Model file for the job. Use its own axes, mm. Face numbers are marked on the shaded views. A direction names the side the tool comes from. Give positions to 0.01 mm unless a question says otherwise; leave off trailing zeros. Order: outer loops, then holes, each group sorted by start corner. A loop starts at its lowest first (then second) coordinate and runs counter-clockwise, first axis right, second up. Notation, with made-up numbers: (58, 8.25) - (106, 8.25) arc R16 ccw to (106, 38.25) - close; hole circle Ø8 at (40, 4). An arc over 180 degrees is marked (long way). Use CSV: the item, a comma, the result in double quotes. Start each with the question number.
(1) Band-saw the part on A-A, the plane x = 0. Count the separate pieces of the cut face and the enclosed holes in it, then the cut area to 3 significant figures.
(2) Probe L1, parallel to Y at x = 0, z = -0.5 (3 decimals); L2, parallel to Y at x = -0.25, z = -3.25 (3 decimals); L3, parallel to Z at x = 4, y = 29. List the from-to ranges inside material, lowest first.
(3) Tool access for the marked faces 1 and 2: list every direction of +Z, -Z, +X, -X, +Y, -Y with a clear straight run to the whole face (end or side of a thin tool).
(4) Band-saw the part on B-B, the plane y = 3. Give the cut face in (x, z).
(5) Drop flat-ended pins along their axis: pin 1 Ø3 at (x, z) = (-1, 2.5) entering from -Y; pin 2 Ø2.5 at (x, z) = (-2, 2) entering from +Y; pin 3 Ø2.5 at (x, y) = (0, 12.065) entering from +Z; pin 4 Ø2 at (x, z) = (-4.76, 0) entering from -Y. Give the stop position or say it passes through.
(6) Band-saw the part on C-C, the plane z = 3.5. Give the cut face in (x, y), then the cut area to 3 significant figures.
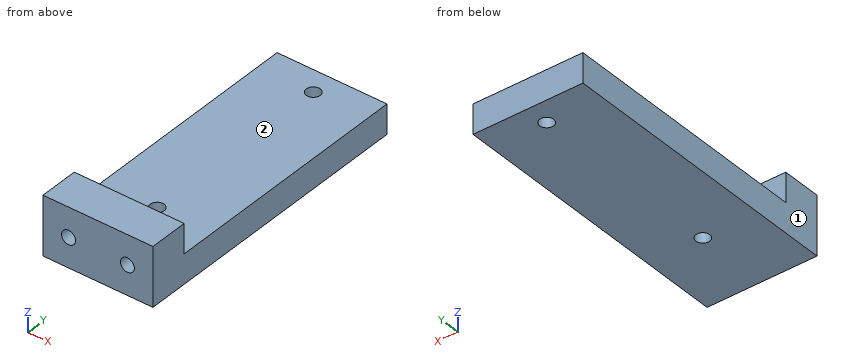
from build123d import *

# Parameters (mm, degrees)
SKETCH1_W                 = 17.78
SKETCH1_H                 = 9.525
BOSS_EXTRUDE1_DEPTH       = 47.625
SKETCH2_W                 = 17.78
SKETCH2_H                 = 4.7625
CUT_EXTRUDE1_DEPTH        = 41.275
F_4_40_TAPPED_HOLE1_D     = 2.2606
F_4_40_TAPPED_HOLE1_DEPTH = 6.35
F_4_40_TAPPED_HOLE1_TIP   = 0.679152758
SKETCH8_R                 = 1.1303
CUT_EXTRUDE2_DEPTH        = 50.375078228


with BuildPart() as part:
    # Sketch1 → Boss-Extrude1 (new body)
    with BuildSketch(Plane(origin=(0, 0, 0), x_dir=(1, 0, 0), z_dir=(0, 1, 0))):
        Rectangle(SKETCH1_W, SKETCH1_H)
    extrude(amount=BOSS_EXTRUDE1_DEPTH)

    # Sketch2 → Cut-Extrude1 (cut)
    with BuildSketch(Plane(origin=(0, 47.625, 0), x_dir=(1, 0, 0), z_dir=(0, 1, 0))):
        with Locations((0, -2.38125)):
            Rectangle(SKETCH2_W, SKETCH2_H)
    extrude(amount=-CUT_EXTRUDE1_DEPTH, mode=Mode.SUBTRACT)

    # #4-40 Tapped Hole1
    with Locations(Plane(origin=(0, 0, 0), x_dir=(-1, 0, 0), z_dir=(0, -1, 0))):
        with Locations((-4.7625, 0), (4.7625, 0)):
            Hole(F_4_40_TAPPED_HOLE1_D / 2, depth=F_4_40_TAPPED_HOLE1_DEPTH)
            with Locations((0, 0, -(F_4_40_TAPPED_HOLE1_DEPTH + F_4_40_TAPPED_HOLE1_TIP / 2))):  # 118° drill point
                Cone(0, F_4_40_TAPPED_HOLE1_D / 2, F_4_40_TAPPED_HOLE1_TIP, mode=Mode.SUBTRACT)

    # Sketch8 → Cut-Extrude2 (cut, through all)
    with BuildSketch(Plane(origin=(0, 0, -4.7625), x_dir=(-1, 0, 0), z_dir=(0, 0, -1))):
        with Locations((0, 43.815)):
            Circle(SKETCH8_R)
        with Locations((0, 12.065)):
            Circle(SKETCH8_R)
    extrude(amount=-CUT_EXTRUDE2_DEPTH, mode=Mode.SUBTRACT)


solid = part.part
Answer block:
1,separate pieces,"3"
1,enclosed holes,"0"
1,area,"236 mm2"
2,L1,"y = 0 to 10.935, 13.195 to 42.685, 44.945 to 47.625"
2,L2,"y = 0 to 10.963, 13.167 to 42.713, 44.917 to 47.625"
2,L3,"z = -4.76 to 0"
3,face 1,"+Z, -Z, -X, +Y, -Y"
3,face 2,"+Z, +X, -X, +Y"
4,outline,"(-8.89, -4.76) - (8.89, -4.76) - (8.89, 4.76) - (-8.89, 4.76) - close; hole circle Ø2.26 at (-4.76, 0); hole circle Ø2.26 at (4.76, 0)"
5,pin 1,"stops at y = 0"
5,pin 2,"stops at y = 6.35"
5,pin 3,"stops at z = 0"
5,pin 4,"stops at y = 6.43"
6,outline,"(-8.89, 0) - (8.89, 0) - (8.89, 6.35) - (-8.89, 6.35) - close"
6,area,"113 mm2"
